Part model, mm, in its own coordinate system. A direction names the side the tool comes from. Give positions to 0.01 mm unless a question says otherwise; leave off trailing zeros. Write each loop counter-clockwise with the first axis right and the second up, starting at its lowest first coordinate (ties: lowest second). Pieces come first, ordered by that corner, then holes. Notation, with made-up numbers: (25, -23.5) - (78, -23.5) arc R18 ccw to (78, -2.5) - close; hole circle Ø8 at (53.25, 58.25). An arc over 180 degrees is marked (long way). Answer in a Markdown table with one row per item. Add a question column.
1. Pull direction X, two halves, no side cores. Call faces 5 (the flat face through (-34, -3.187, -1)), 6 (the flat face through (-34.65, -8, -1)), 7 (the cylindrical face through (-34.67, 23.31, 1.36)), 8 (the flat face through (39.75, -13, 1)): released by +X, released by -X, zero draft, split by the parting line, or undercut.
2. Band-saw the part on A-A on y = 15.5. Write the cut outline in (x, z), plus the area to 3 significant figures.
3. Band-saw the part on B-B on z = -1.1. Write the cut outline in (x, y) (3 decimals), plus the area to 3 significant figures.
4. Band-saw the part on D-D on y = -14. Write the cut outline in (x, z), plus the area to 3 significant figures.
5. Drop flat-ended pins along their axis: pin 1 Ø0.8 at (x, y) = (-34.5, -8.5) entering from -Z; pin 2 Ø2.5 at (y, z) = (-7, -1.5) entering from -X; pin 3 Ø1.4 at (x, z) = (3, -2) entering from -Y; pin 4 Ø4 at (x, y) = (34.85, -22.39) entering from +Z. Give the stop position or say it passes through.
6. Band-saw the part on C-C on x = 15. Write the cut outline in (y, z), plus the area to 3 significant figures.
7. Which spindle directions (+Z, -Z, +X, -X, +Y, -Y) get a long thin tool onto all of the face, cutting with end or side? Do faces 1 (the flat face through (-1, -14.987, -1)), 2 (the flat face through (10.287, 5.055, -1.38)), 3 (the flat face through (34, 4, -2.3)), 4 (the flat face through (20, -5.237, 2)). Say none if no direction does.
8. Probe line 1 along Y through (x, z) = (0, 0.8); line 2 along Y through (x, z) = (0, -0.1); line 3 along Y through (x, z) = (2.5, -0.9). List the from-to ranges inside material, lowest first.
Autodesk Inventor part; units mm, degrees
ref_plane "YZ Plane" through (0, 0, 0) normal (1, 0, 0) x (0, 1, 0)
ref_plane "XZ Plane" through (0, 0, 0) normal (0, 1, 0) x (-1, 0, 0)
ref_plane "XY Plane" through (0, 0, 0) normal (0, 0, 1) x (1, 0, 0)
sketch "Sketch1" plane through (0, 0, 0) normal (0, 0, 1) x (1, 0, 0)
  line L0 (-8.76, 11.0126) -> (-8.76, 0.5126)
  line L1 (-8.76, 0.5126) -> (-11.24, -14.9874)
  line L2 (-11.24, -14.9874) -> (8.76, -14.9874)
  line L3 (8.76, -14.9874) -> (8.76, -4.4874)
  line L4 (11.24, 11.0126) -> (-8.76, 11.0126)
  line L5 (0, 12.916) -> (0, -18.5653)
  line L6 (-8.76, 0.5126) -> (13.6474, 0.5126) construction
  line L7 (8.76, -4.4874) -> (-2.6872, -4.4874) construction
  line L8 (-5.8361, -1.9874) -> (18.6079, -1.9874) construction
  circle A0 centre (0, -7.7374) radius 1.325
  circle A1 centre (0, 3.7626) radius 1.325
  line L9 (22.7948, -1.9874) -> (0, -1.9874) construction
  line L10 (9.36, -0.7374) -> (0, -0.7374)
  line L11 (0, -3.2374) -> (8.96, -3.2374)
  arc A2 (0, -0.7374) -> (0, -3.2374) centre (0, -1.9874) ccw
  line L12 (8.76, -4.4874) -> (8.96, -3.2374)
  line L13 (9.36, -0.7374) -> (11.24, 11.0126)
  point P0 (0, 0)
  point P1 (-8.76, -4.4874)
  point P2 (11.3974, -1.9874)
  dimension "d0" = 2.48
  dimension "d1" = 15.5
  dimension "d2" = 15.5
  dimension "d3" = 2.48
  dimension "d4" = 10.5
  dimension "d5" = 10.5
  dimension "d6" = 20
  dimension "d7" = 20
  dimension "d8" = 2.65
  dimension "d9" = 7.25
  dimension "d12" = 2.5
  dimension "d26" = 11.75
  dimension "d27" = 14.25
extrude "Extrusion1" add sketch "Sketch1" against normal blind 2.8 contours L4 L5 A1 A2 A0 L2 L1 L0 | L4 L13 L10 L5 A1 | L5 A0 L11 L12 L3 L2
sketch "Sketch2" plane through (0, 0, 0) normal (0, 0, 1) x (1, 0, 0)
  line L0 (-39.75, -18.5874) -> (-39.75, 14.6126)
  line L1 (0, 12.916) -> (0, -18.5653) construction
  line L2 (-5.8361, -1.9874) -> (18.6079, -1.9874) construction
  line L3 (-39.75, 14.6126) -> (-39.75, 18.4126)
  line L4 (-29.9847, 14.6126) -> (-29.9847, 17.8301)
  arc A0 (-29.9847, 17.8301) -> (-39.75, 18.4126) centre (-34.85, 18.4126) ccw
  line L5 (0, 12.916) -> (0, -18.5653)
  circle A1 centre (-34.85, 18.4126) radius 2.1
  arc A2 (0, -0.7374) -> (0, -3.2374) centre (0, -1.9874) ccw
  line L6 (-1.25, -1.9874) -> (17.7749, -1.9874) construction
  line L7 (0, -3.2374) -> (39.75, -3.2374)
  line L8 (39.75, -0.7374) -> (0, -0.7374)
  arc A3 (0, -0.7374) -> (0, -3.2374) centre (0, -1.9874) ccw
  line L9 (39.75, 14.6126) -> (39.75, -0.7374)
  line L10 (39.75, -3.2374) -> (39.75, -18.5874)
  line L11 (27.8114, -18.5874) -> (2.6919, -18.5874)
  line L12 (29.9847, -18.5874) -> (-29.9847, -18.5874)
  circle A4 centre (0, 3.7626) radius 1.325
  circle A5 centre (0, -7.7374) radius 1.325
  line L13 (-29.9847, 14.6126) -> (29.9847, 14.6126)
  line L14 (39.75, 14.6126) -> (39.75, 18.4126)
  line L15 (29.9847, 14.6126) -> (29.9847, 17.8301)
  arc A6 (39.75, 18.4126) -> (29.9847, 17.8301) centre (34.85, 18.4126) ccw
  circle A7 centre (34.85, 18.4126) radius 2.1
  line L16 (-39.75, -18.5874) -> (-39.75, -22.3874)
  line L17 (-29.9847, -18.5874) -> (-29.9847, -21.8049)
  arc A8 (-39.75, -22.3874) -> (-29.9847, -21.8049) centre (-34.85, -22.3874) ccw
  circle A9 centre (-34.85, -22.3874) radius 2.1
  line L18 (29.9847, -18.5874) -> (29.9847, -21.8049)
  circle A10 centre (34.85, -22.3874) radius 2.1
  line L19 (39.75, -18.5874) -> (39.75, -22.3874)
  arc A11 (29.9847, -21.8049) -> (39.75, -22.3874) centre (34.85, -22.3874) ccw
  point P0 (0, 0)
  point P1 (8.2624, -1.9874)
  point P2 (27.8114, 14.6126)
  dimension "d15" = 4.9
  dimension "d16" = 4.2
  dimension "d25" = 79.5
extrude "Extrusion2" add sketch "Sketch2" along normal blind 2.75 contours L0 L3 A0 L4 L13 L15 A6 L14 L9 L8 A2 L7 L10 L19 A11 L18 L12 L11 L17 A8 L16
sketch "Sketch3" plane through (0, 0, 2.75) normal (0, 0, 1) x (1, 0, 0)
  arc A0 (0, -0.7374) -> (0, -3.2374) centre (0, -1.9874) ccw
  line L0 (0, -1.9874) -> (45.1297, -1.9874) construction
  line L1 (0, -5.2374) -> (45.1297, -5.2374)
  line L2 (45.1297, 1.2626) -> (0, 1.2626)
  arc A1 (0, 1.2626) -> (0, -5.2374) centre (0, -1.9874) ccw
  arc A2 (45.1297, -5.2374) -> (45.1297, 1.2626) centre (45.1297, -1.9874) ccw
  point P0 (0, 0)
  point P1 (22.5649, -1.9874)
  dimension "d20" = 3.25
extrude "Extrusion3" cut sketch "Sketch3" against normal blind 1.65
sketch "Sketch4" plane through (0, 0, 0) normal (0, 0, -1) x (-1, 0, 0)
  line L0 (-34.65, 8.0126) -> (-33.15, 8.0126)
  line L1 (-33.15, 8.0126) -> (-33.15, -0.7874)
  line L2 (-33.15, -0.7874) -> (-34.65, -0.7874)
  line L3 (-34.65, -0.7874) -> (-34.65, 8.0126)
  line L4 (-39.75, -0.7374) -> (-39.75, 18.4126)
  line L5 (-29.9847, 14.6126) -> (29.9847, 14.6126)
  line L6 (33.15, -3.1874) -> (34.65, -3.1874)
  line L7 (34.65, -3.1874) -> (34.65, -11.9874)
  line L8 (34.65, -11.9874) -> (33.15, -11.9874)
  line L9 (33.15, -11.9874) -> (33.15, -3.1874)
  line L10 (39.75, 18.4126) -> (39.75, -22.3874)
  line L11 (29.9847, -18.5874) -> (-29.9847, -18.5874)
  point P0 (0, 0)
  point P1 (-39.75, 8.8376)
  dimension "d28" = 5.1
  dimension "d29" = 6.6
  dimension "d30" = 8.8
  dimension "d31" = 1.5
  dimension "d32" = 5.1
  dimension "d33" = 6.6
  dimension "d34" = 8.8
  dimension "d35" = 1.5
extrude "Extrusion4" add sketch "Sketch4" along normal blind 2.3
properties part number "Gripper_BackPlate"
Values:
| question | item | result |
|---|---|---|
| 1 | face 5 | zero draft |
| 1 | face 6 | released by -X |
| 1 | face 7 | undercut |
| 1 | face 8 | released by +X |
| 2 | outline | (-39.75, 0) - (-29.98, 0) - (-29.98, 2.75) - (-39.75, 2.75) - close; (29.98, 0) - (39.75, 0) - (39.75, 2.75) - (29.98, 2.75) - close |
| 2 | area | 53.7 mm² |
| 3 | outline | (-34.65, -11.987) - (-33.15, -11.987) - (-33.15, -3.187) - (-34.65, -3.187) - close; (-11.24, -14.987) - (8.76, -14.987) - (8.76, -4.487) - (8.96, -3.237) - (0, -3.237) arc R1.25 cw to (0, -0.737) - (9.36, -0.737) - (11.24, 11.013) - (-8.76, 11.013) - (-8.76, 0.513) - close; (33.15, -0.787) - (34.65, -0.787) - (34.65, 8.013) - (33.15, 8.013) - close; hole circle Ø2.65 at (0, -7.737); hole circle Ø2.65 at (0, 3.763) |
| 3 | area | 484 mm² |
| 4 | outline | (-39.75, 0) - (-11.08, 0) - (-11.08, -2.8) - (8.76, -2.8) - (8.76, 0) - (39.75, 0) - (39.75, 2.75) - (-39.75, 2.75) - close |
| 4 | area | 274 mm² |
| 5 | pin 1 | stops at z = -2.3 |
| 5 | pin 2 | stops at x = -34.65 |
| 5 | pin 3 | stops at y = -14.99 |
| 5 | pin 4 | passes through |
| 6 | outline | (-18.59, 0) - (-3.24, 0) - (-3.24, 1.1) - (-5.24, 1.1) - (-5.24, 2.75) - (-18.59, 2.75) - close; (-0.74, 0) - (14.61, 0) - (14.61, 2.75) - (1.26, 2.75) - (1.26, 1.1) - (-0.74, 1.1) - close |
| 6 | area | 77.8 mm² |
| 7 | face 1 | -Z, +X, -X, -Y |
| 7 | face 2 | -Z, -Y |
| 7 | face 3 | -Z, +X, +Y, -Y |
| 7 | face 4 | +Z, +X |
| 8 | line 1 | y = -18.59 to -9.06, -6.41 to -3.24, -0.74 to 2.44, 5.09 to 14.61 |
| 8 | line 2 | y = -14.99 to -9.06, -6.41 to -3.24, -0.74 to 2.44, 5.09 to 11.01 |
| 8 | line 3 | y = -14.99 to -3.24, -0.74 to 11.01 |
